from build123d import *

# Parameters (mm, degrees)
SKETCH_2_R                   = 25
EXTRUDE_2_DEPTH              = 2
SKETCH_22_R                  = 10
CUT_EXTRUDE_1_DEPTH          = 2
FILLET_4_R                   = 0.2
SKETCH_54_R                  = 25
EXTRUDE_6_DEPTH              = 10
SKETCH_55_R                  = 18.5
CUT_EXTRUDE_2_DEPTH          = 8
HOLE_WIZARD_M4_1_D           = 4.5
HOLE_WIZARD_M4_1_CBORE_D     = 8
HOLE_WIZARD_M4_1_CBORE_DEPTH = 1
PATTERN_CIRCULAR_1_COUNT     = 3
SKETCH_59_R                  = 18.5
SKETCH_59_R_2                = 17.5
EXTRUDE_7_DEPTH              = 1
EXTRUDE_8_DEPTH              = 9
FILLET_6_R                   = 0.3
SKETCH_68_R                  = 9.5
CUT_EXTRUDE_7_DEPTH          = 7
SKETCH_69_R                  = 8.5
CUT_EXTRUDE_8_DEPTH          = 3
FILLET_7_R                   = 0.3


with BuildPart() as part:
    # 스케치2 → 보스-돌출2 (new body)
    with BuildSketch(Plane(origin=(0, 6, 0), x_dir=(1, 0, 0), z_dir=(0, 0, -1))):
        with Locations((0, 6)):
            Circle(SKETCH_2_R)
    extrude(amount=EXTRUDE_2_DEPTH)

    # 스케치22 → 컷-돌출1 (cut)
    with BuildSketch(Plane.XY):
        Circle(SKETCH_22_R)
    extrude(amount=-CUT_EXTRUDE_1_DEPTH, mode=Mode.SUBTRACT)

    # 필렛4
    fillet_4_edges = [part.edges().sort_by_distance(p)[0] for p in [
        (-10, 0, 0),
    ]]
    fillet(fillet_4_edges, radius=FILLET_4_R)

    # 스케치54 → 보스-돌출6 (add)
    with BuildSketch(Plane(origin=(0, 0, -2), x_dir=(-1, 0, 0), z_dir=(0, 0, -1))):
        Circle(SKETCH_54_R)
    extrude(amount=EXTRUDE_6_DEPTH)

    # 스케치55 → 컷-돌출2 (cut)
    with BuildSketch(Plane(origin=(0, 0, -12), x_dir=(-1, 0, 0), z_dir=(0, 0, -1))):
        Circle(SKETCH_55_R)
    extrude(amount=-CUT_EXTRUDE_2_DEPTH, mode=Mode.SUBTRACT)

    # M4 육각 소켓 머리 캡 나사용 카운터보어1 (through all)
    with Locations(Plane(origin=(0, 0, -4), x_dir=(-1, 0, 0), z_dir=(0, 0, -1))):
        with Locations((0, 6)):
            hole_wizard_m4_1 = CounterBoreHole(HOLE_WIZARD_M4_1_D / 2, HOLE_WIZARD_M4_1_CBORE_D / 2, HOLE_WIZARD_M4_1_CBORE_DEPTH)

    # 원형 패턴1: M4 육각 소켓 머리 캡 나사용 카운터보어1 ×3 about axis
    pattern_circular_1_axis = Axis((0, 0, 0), (0, 0, 1))
    for i in range(1, PATTERN_CIRCULAR_1_COUNT):
        add(hole_wizard_m4_1.rotate(pattern_circular_1_axis, i * 360 / PATTERN_CIRCULAR_1_COUNT), mode=Mode.SUBTRACT)

    # 스케치59 → 보스-돌출7 (add)
    with BuildSketch(Plane(origin=(0, 0, -4), x_dir=(-1, 0, 0), z_dir=(0, 0, -1))):
        Circle(SKETCH_59_R)
        Circle(SKETCH_59_R_2, mode=Mode.SUBTRACT)
    extrude(amount=EXTRUDE_7_DEPTH)

    # 스케치60 → 보스-돌출8 (add)
    with BuildSketch(Plane(origin=(0, 0, -12), x_dir=(-1, 0, 0), z_dir=(0, 0, -1))):
        with BuildLine():
            Line((-24.65033243, -4.166666667), (-14.790199458, -62.5))
            ThreePointArc((-14.790199458, -62.5), (0, -75), (14.790199458, -62.5))
            Line((14.790199458, -62.5), (24.65033243, -4.166666667))
            ThreePointArc((24.65033243, -4.166666667), (0, -25), (-24.65033243, -4.166666667))
        make_face()
    extrude(amount=-EXTRUDE_8_DEPTH)

    # 필렛6
    fillet_6_edges = [part.edges().sort_by_distance(p)[0] for p in [
        (18.5, 0, -5),
    ]]
    fillet(fillet_6_edges, radius=FILLET_6_R)

    # 스케치68 → 컷-돌출7 (cut)
    with BuildSketch(Plane.XY.offset(-3)):
        with Locations((0, -60)):
            Circle(SKETCH_68_R)
    extrude(amount=-CUT_EXTRUDE_7_DEPTH, mode=Mode.SUBTRACT)

    # 스케치69 → 컷-돌출8 (cut, through all)
    with BuildSketch(Plane.XY.offset(-10)):
        with Locations((0, -60)):
            Circle(SKETCH_69_R)
    extrude(amount=-CUT_EXTRUDE_8_DEPTH, mode=Mode.SUBTRACT)

    # 필렛7
    fillet_7_edges = [part.edges().sort_by_distance(p)[0] for p in [
        (-9.5, -60, -10),
    ]]
    fillet(fillet_7_edges, radius=FILLET_7_R)


solid = part.part
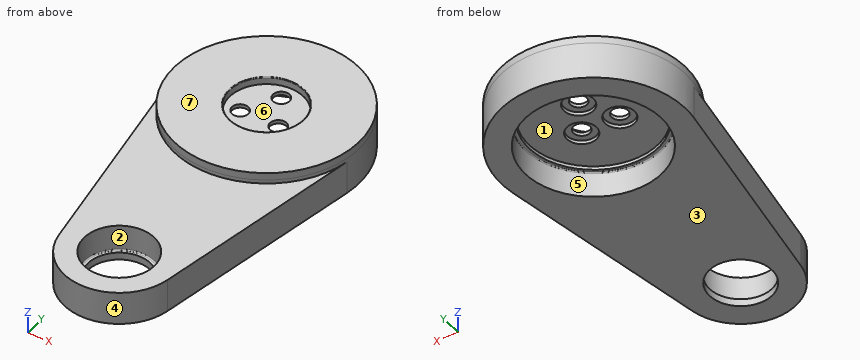
Geometry: final body of the model. Coordinates: model frame, mm. Face numbers are marked on the shaded views. A direction names the side the tool comes from. Give positions to 0.01 mm unless a question says otherwise; leave off trailing zeros. Write each loop counter-clockwise with the first axis right and the second up, starting at its lowest first coordinate (ties: lowest second). Pieces come first, ordered by that corner, then holes.
(1) Access query for the marked faces 1, 2 and 3. Directions: +Z, -Z, +X, -X, +Y, -Y. A direction counts if a zero-diameter tool reaches every point of the face in a straight line with its end or side. Return the directions, or none.
(2) Mould query, pull axis Y, two halves, no side actions, for the marked faces 4, 5, 6 and 7. Classes: released by +Y, released by -Y, zero draft, split by the parting line, or undercut.
(3) Cut plane B-B, the plane x = 0. Give the number of separate pieces and of enclosed holes in the cut face, then the cut area to 3 significant figures.
(4) Ray query, line 1 (Y direction, x = 7, z = -6); line 2 (Y direction, x = -2.5, z = -3.5); line 3 (Y direction, x = 0, z = -0.7). Return the intervals inside material, ascending.
(5) First-contact query: P1, Ø5, axis at x = 5.2, y = -3, coming from the +Z side; P2, Ø22, axis at x = 0, y = -60, coming from the +Z side; P3, Ø12, axis at x = 2.5, y = 4.5, coming from the -Z side; P4, Ø2.5, axis at x = -5.2, y = -3, coming from the -Z side. Flat tips, straight axial feed; report the tip coordinate or a pass-through.
(6) Cut plane C-C, the plane y = -45. Return loops of the section in (x, z), then the cut area to 3 significant figures.
(7) Cut plane A-A, the plane z = -8.5. Return loops of the section in (x, y).
Values follow:
1. face 1: -Z
1. face 2: +Z
1. face 3: -Z, +X, -X, +Y, -Y
2. face 4: released by -Y
2. face 5: undercut
2. face 6: undercut
2. face 7: zero draft
3. separate pieces: 3
3. enclosed holes: 0
3. area: 537 mm2
4. line 1: y = -73.27 to -66.42, -53.58 to -17.12, 17.12 to 24
4. line 2: y = -74.79 to -69.17, -50.83 to -5.95, -0.05 to 2.88, 9.12 to 24.87
4. line 3: y = -25 to -10, 10 to 25
5. P1: stops at z = -2
5. P2: stops at z = -3
5. P3: stops at z = -4
5. P4: passes through
6. outline: (-17.75, -12) - (17.75, -12) - (17.75, -3) - (-17.75, -3) - close
6. area: 319 mm2
7. outline: (-24.65, -4.17) - (-14.79, -62.5) arc R15 ccw to (14.79, -62.5) - (24.65, -4.17) arc R25 ccw (long way) to start; hole circle Ø37 at (0, 0); hole circle Ø19 at (0, -60)
